Build history of the part. All positions in model axes, mm. Give positions to 0.01 mm unless a question says otherwise; leave off trailing zeros. Loops run counter-clockwise (first coordinate to the right, second up) from the corner with the lowest first, then second, coordinate; pieces in that order, holes last. Notation, with made-up numbers: M -29.75,33 L 15.25,33 A29 ccw 15.25,59 Z; hole C 87.25,83.25 d10. An arc over 180 degrees is marked long. Put each result on its own line as item: value.
```python
from build123d import *

# Parameters (mm, degrees)
F1_DEPTH = 25.4


with BuildPart() as f1:
    # F0 (on Top) → F1 (new body)
    with BuildSketch(Plane.XY):
        with BuildLine():
            Line((0, 25.4), (0, 0))
            Line((0, 0), (28.306466, 0))
            Line((28.306466, 0), (28.306466, 25.4))
            Line((28.306466, 25.4), (20.503233, 25.4))
            ThreePointArc((20.503233, 25.4), (14.153233, 19.05), (7.803233, 25.4))
            Line((7.803233, 25.4), (0, 25.4))
        make_face()
        with BuildLine():
            ThreePointArc((28.306466, 25.4), (14.153233, 39.553233), (0, 25.4))
            Line((0, 25.4), (7.803233, 25.4))
            ThreePointArc((7.803233, 25.4), (14.153233, 31.75), (20.503233, 25.4))
            Line((20.503233, 25.4), (28.306466, 25.4))
        make_face()
    extrude(amount=F1_DEPTH)


solid = f1.part
```
Q1. Slice it at A-A (x = 17.75). List the corners of the cut face in (y, z).
Here are the results:
outline: M 0,0 L 20.17,0 L 20.17,25.4 L 0,25.4 Z; M 30.63,0 L 39.09,0 L 39.09,25.4 L 30.63,25.4 Z
Q2. Mould opens along Y. For faces 1 (the flat face through (14, 0, 13)), 2 (the cylindrical face through (14.46, 39.55, 12.52)), 3 (the flat face through (14, 16, 0)), 4 (the cylindrical face through (11.22, 19.77, 12.52)) say: pulls with the +Y half, pulls with the -Y half, needs draft (parallel to the pull), parting line crosses it, or undercut.
Here are the results:
face 1: pulls with the -Y half
face 2: pulls with the +Y half
face 3: needs draft
face 4: undercut
Q3. Slice it at C-C (z = 16). List the corners of the cut face in (x, y).
Here are the results:
outline: M 0,0 L 28.31,0 L 28.31,25.4 A14.15 ccw 0,25.4 Z; hole C 14.15,25.4 d12.7
Q4. Drop flat-ended pins along their axis: pin 1 Ø12 at (x, z) = (20.5, 16.5) entering from +Y; pin 2 Ø10 at (x, y) = (14.15, 25.4) entering from +Z; pin 3 Ø10 at (y, z) = (34, 14) entering from +X; pin 4 Ø6 at (x, z) = (23, 9.5) entering from +Y. Give the stop position or say it passes through.
Here are the results:
pin 1: y = 39.55
pin 2: through
pin 3: x = 27.84
pin 4: y = 38.29
Q5. Probe line 1 (Y direction, x = 18.25, z = 15); line 2 (Y direction, x = 13.75, z = 15.5); line 3 (Y direction, x = 21.75, z = 8). List the from-to ranges inside material, lowest first. Write a range as from..to.
Here are the results:
line 1: 0..20.55, 30.25..38.95
line 2: 0..19.06, 31.74..39.55
line 3: 0..37.34
Q6. Slice it at D-D (y = 36.5). List the corners of the cut face in (x, z), and give its area (3 significant figures).
Here are the results:
outline: M 5.37,0 L 22.93,0 L 22.93,25.4 L 5.37,25.4 Z
area: 446 mm²
Q7. Slice it at B-B (y = 30.5). List the corners of the cut face in (x, z).
Here are the results:
outline: M 0.95,0 L 10.37,0 L 10.37,25.4 L 0.95,25.4 Z; M 17.94,0 L 27.36,0 L 27.36,25.4 L 17.94,25.4 Z
